from build123d import *

# Parameters (mm, degrees)
F1_DEPTH = 40
F2_R     = 20
F4_DEPTH = 18.572422
F5_R     = 7.5
F6_DEPTH = 16.624377


with BuildPart() as f1:
    # F0 (on Right) → F1 (new body, symmetric)
    with BuildSketch(Plane.YZ):
        with BuildLine():
            Line((-63.67937, -21.339411), (-110.237809, -21.339411))
            Line((-110.237809, -21.339411), (-110.237809, -37.962787))
            Line((-110.237809, -37.962787), (-50.237809, -37.962787))
            ThreePointArc((-50.237809, -37.962787), (-25.237809, -12.962787), (-0.237809, -37.962787))
            Line((-0.237809, -37.962787), (84.762191, -37.962787))
            Line((84.762191, -37.962787), (84.762191, 43.595657))
            Line((84.762191, 43.595657), (66.190769, 43.595657))
            Line((66.190769, 43.595657), (66.190769, -21.339411))
            Line((66.190769, -21.339411), (13.203752, -21.339411))
            ThreePointArc((13.203752, -21.339411), (-25.237809, 3.919073), (-63.67937, -21.339411))
        make_face()
    extrude(amount=F1_DEPTH, both=True)

    # F2
    f2_edges = [f1.edges().sort_by_distance(p)[0] for p in [
        (40, -110.237809, -29.651099),
        (-40, -110.237809, -29.651099),
        (40, 75.47648, 43.595657),
        (-40, 75.47648, 43.595657),
    ]]
    fillet(f2_edges, radius=F2_R)

    # F3 (on face) → F4 (cut, through all)
    with BuildSketch(Plane.XZ.offset(-66.190769)):
        with BuildLine():
            Line((-7, 43.595657), (-7, 20))
            ThreePointArc((-7, 20), (0, 13), (7, 20))
            Line((7, 20), (7, 43.595657))
            Line((7, 43.595657), (-7, 43.595657))
        make_face()
    extrude(amount=-F4_DEPTH, mode=Mode.SUBTRACT)

    # F5 (on face) → F6 (cut, through all)
    with BuildSketch(Plane.XY.offset(-21.339411)):
        with Locations((-20, -90.237809)):
            Circle(F5_R)
        with Locations((20, -90.237809)):
            Circle(F5_R)
    extrude(amount=-F6_DEPTH, mode=Mode.SUBTRACT)


solid = f1.part
Source: CAD feature listing. Evaluate the final solid. Frame: model axes, mm. A direction names the side the tool comes from. Round coordinates to 2 decimals unless told otherwise and drop trailing zeros. Loops run counter-clockwise (first coordinate to the right, second up) from the corner with the lowest first, then second, coordinate; pieces in that order, holes last. Notation, with made-up numbers: M 53.5,21.5 L 66.5,21.5 A21 cw 66.5,50.5 Z; hole C -9.75,68.5 d4. An arc over 180 degrees is marked long. Answer as CSV lines item,"result".
Q1. Cut plane B-B (x = 0). Return the cut outline in (y, z).
Verdict:
outline,"M -110.24,-37.96 L -50.24,-37.96 A25 cw -0.24,-37.96 L 84.76,-37.96 L 84.76,13 L 66.19,13 L 66.19,-21.34 L 13.2,-21.34 A41.88 ccw -63.68,-21.34 L -110.24,-21.34 Z"
Q2. Cut plane A-A (z = -29). Return the cut outline in (x, y).
Verdict:
outline,"M -40,-90.24 A20 ccw -20,-110.24 L 20,-110.24 A20 ccw 40,-90.24 L 40,-48.58 L -40,-48.58 Z; M -40,-1.9 L 40,-1.9 L 40,84.76 L -40,84.76 Z; hole C -20,-90.24 d15; hole C 20,-90.24 d15"
Q3. Contact query for flat-ended pins moving along their axis: pin 1 (9 mm diameter, centred on x = -20, y = -90.24, fed in from +Z); pin 2 (6 mm diameter, centred on x = -31.5, z = 13, fed in from -Y); pin 3 (6 mm diameter, centred on x = -8, y = 43.5, fed in from +Z); pin 4 (8 mm diameter, centred on x = -9.5, y = -42, fed in from +Z). Output: stop coordinate, or through.
Verdict:
pin 1,"passes through"
pin 2,"stops at y = 66.19"
pin 3,"stops at z = -21.34"
pin 4,"stops at z = 1.93"
Q4. Reachability of faces 4 (the face through (1, 84.762, 2)), 5 (the face through (-7, 75, 32)), 6 (the face through (1, 40, -21.339)) from +Z, -Z, +X, -X, +Y, -Y: full face, straight path, thin tool, end or side. Return the list, or none.
Verdict:
face 4,"+Z, -Z, +X, -X, +Y"
face 5,"+Z, +Y, -Y"
face 6,"+Z, +X, -X"
Q5. Cut plane C-C (z = 38.5). Return the cut outline in (x, y), plus the area to 3 significant figures.
Verdict:
outline,"M -33.34,66.19 L -7,66.19 L -7,84.76 L -33.34,84.76 Z; M 7,66.19 L 33.34,66.19 L 33.34,84.76 L 7,84.76 Z"
area,"978 mm^2"
Q6. Pull-direction query (Y, two-part tool) for faces 1 (the face through (-25.53, -85.17, -29.53)), 2 (the face through (7, 75, 32)), 3 (the face through (34.3, -104.22, -29.77)); classes: +Y half, -Y half, draft (parallel to the pull), parting line (faces both ways), or undercut.
Verdict:
face 1,"undercut"
face 2,"draft"
face 3,"-Y half"
Q7. Line query: line 1 along Y through (x, z) = (-20, -31); line 2 along Y through (x, z) = (-20, -28); line 3 along Z through (x, y) = (7.5, 55). Output: solid intervals per line, ascending.
Verdict:
line 1,"y = -110.24 to -97.74, -82.74 to -49.25, -1.23 to 84.76"
line 2,"y = -110.24 to -97.74, -82.74 to -48.17, -2.31 to 84.76"
line 3,"z = -37.96 to -21.34"
Q8. Cut plane D-D (y = 31). Return the cut outline in (x, z), plus the area to 3 significant figures.
Verdict:
outline,"M -40,-37.96 L 40,-37.96 L 40,-21.34 L -40,-21.34 Z"
area,"1,330 mm^2"
